CAD build for the part. Positions are in the model's coordinates, mm. Face numbers are marked on the shaded views. A direction names the side the tool comes from. Round coordinates to 2 decimals unless told otherwise and drop trailing zeros. Loops run counter-clockwise (first coordinate to the right, second up) from the corner with the lowest first, then second, coordinate; pieces in that order, holes last. Notation, with made-up numbers: (-8.5, 25.5) - (4.5, 25.5) arc R17 cw to (4.5, 52.5) - close; hole circle Ø10 at (55.5, 52). An arc over 180 degrees is marked (long way). One line per question, with ' | ' between items.
```python
from build123d import *

# Parameters (mm, degrees)
SKETCH1_R           = 12
BOSS_EXTRUDE1_DEPTH = 2
SKETCH2_R           = 12
BOSS_EXTRUDE2_DEPTH = 1
SKETCH3_R           = 6
BOSS_EXTRUDE3_DEPTH = 2.2
SKETCH4_R           = 3
CUT_EXTRUDE1_DEPTH  = 2.6
CUT_EXTRUDE2_REACH  = 19.583
SKETCH5_R           = 1.25
CHAMFER1_SIZE       = 0.2


with BuildPart() as part:
    # Sketch1 → Boss-Extrude1 (new body)
    with BuildSketch(Plane(origin=(0, 0, 0), x_dir=(1, 0, 0), z_dir=(0, 1, 0))):
        with Locations(Location((0, 0, 0), (0, 0, 270))):
            Circle(SKETCH1_R)
        Polygon((-4.907477288, -8.5), (4.907477288, -8.5), (9.814954576, 0), (4.907477288, 8.5), (-4.907477288, 8.5), (-9.814954576, 0), align=None, mode=Mode.SUBTRACT)
    extrude(amount=BOSS_EXTRUDE1_DEPTH)

    # Sketch2 → Boss-Extrude2 (add)
    with BuildSketch(Plane(origin=(0, 2, 0), x_dir=(1, 0, 0), z_dir=(0, 1, 0))):
        with Locations(Location((0, 0, 0), (0, 0, 270))):
            Circle(SKETCH2_R)
    extrude(amount=BOSS_EXTRUDE2_DEPTH)

    # Sketch3 → Boss-Extrude3 (add)
    with BuildSketch(Plane(origin=(0, 3, 0), x_dir=(1, 0, 0), z_dir=(0, 1, 0))):
        with Locations(Location((0, 0, 0), (0, 0, 270))):
            Circle(SKETCH3_R)
    extrude(amount=BOSS_EXTRUDE3_DEPTH)

    # Sketch4 → Cut-Extrude1 (cut)
    with BuildSketch(Plane.XZ.offset(-2)):
        with Locations(Location((0, 0, 0), (0, 0, 270))):
            Circle(SKETCH4_R)
    extrude(amount=-CUT_EXTRUDE1_DEPTH, mode=Mode.SUBTRACT)

    # Sketch5 → Cut-Extrude2 (cut, up to next)
    with BuildSketch(Plane.XZ.offset(-4.6), mode=Mode.PRIVATE) as cut_extrude2_sk1:
        with Locations(Location((0, 0, 0), (0, 0, 270))):
            Circle(SKETCH5_R)
    cut_extrude2_tool1 = extrude(cut_extrude2_sk1.sketch, amount=-CUT_EXTRUDE2_REACH, mode=Mode.PRIVATE) & part.part
    add(cut_extrude2_tool1.solids().sort_by_distance((0, 4.6, 0))[0], mode=Mode.SUBTRACT)

    # Chamfer1
    chamfer1_edges = [part.edges().sort_by_distance(p)[0] for p in [
        (0, 3, -12),
        (0, 5.2, -6),
    ]]
    chamfer(chamfer1_edges, length=CHAMFER1_SIZE)


solid = part.part
```
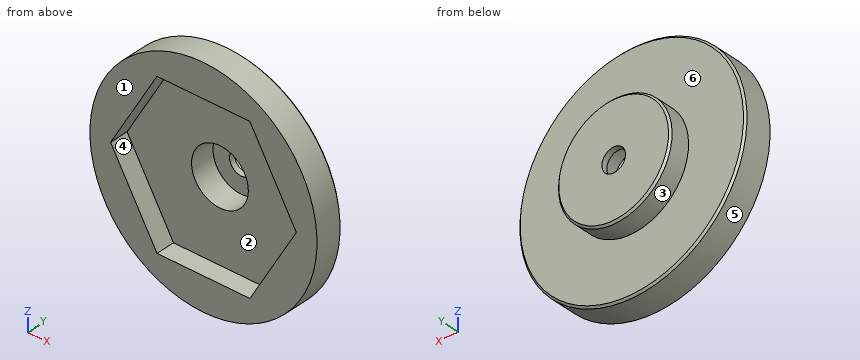
(1) Cut at C-C, the plane y = 2.35. Write the cut outline in (x, z).
Results found:
outline: circle Ø24 at (0, 0); hole circle Ø6 at (0, 0)
(2) Cut at B-B, the plane x = 0. Write the cut outline in (y, z), then the cut area to 3 significant figures.
Results found:
outline: (0, -12) - (2.8, -12) - (3, -11.8) - (3, -6) - (5, -6) - (5.2, -5.8) - (5.2, -1.25) - (4.6, -1.25) - (4.6, -3) - (2, -3) - (2, -8.5) - (0, -8.5) - close; (0, 8.5) - (2, 8.5) - (2, 3) - (4.6, 3) - (4.6, 1.25) - (5.2, 1.25) - (5.2, 5.8) - (5, 6) - (3, 6) - (3, 11.8) - (2.8, 12) - (0, 12) - close | area: 47.2 mm²
(3) Cut at A-A, the plane y = 0.7. Write the cut outline in (x, z), then the cut area to 3 significant figures.
Results found:
outline: circle Ø24 at (0, 0); hole (-9.81, 0) - (-4.91, -8.5) - (4.91, -8.5) - (9.81, 0) - (4.91, 8.5) - (-4.91, 8.5) - close | area: 202 mm²
(4) Probe L1, parallel to Y at x = 3.75, z = -1.5; L2, parallel to Z at x = -5.25, y = 1.7; L3, parallel to Y at x = 8, z = 5.5. List the from-to ranges inside material, lowest first.
Results found:
L1: y = 2 to 5.2 | L2: z = -10.79 to -7.91, 7.91 to 10.79 | L3: y = 0 to 3
(5) Two-plate mould, pull along Z, no slides. Class the marked faces 1, 2 and 3: released by +Z, released by -Z, zero draft, split by the parting line, or undercut.
Results found:
face 1: zero draft | face 2: undercut | face 3: split by the parting line
(6) Drop flat-ended pins along their axis: P1, Ø1.6, axis at x = -2, y = 1, coming from the +Z side; P2, Ø1.5, axis at y = 3.5, z = -7.5, coming from the +X side; P3, Ø1, axis at y = 1, z = -4, coming from the +X side. Give the stop position or say it passes through.
Results found:
P1: stops at z = 11.94 | P2: stops at x = 9.59 | P3: stops at x = 11.48
(7) Tool access for the marked faces 4, 5 and 6: list every direction of +Z, -Z, +X, -X, +Y, -Y with a clear straight run to the whole face (end or side of a thin tool).
Results found:
face 4: -Y | face 5: +Y, -Y | face 6: +Y
